Design review of the part built by this model. Coordinates are the model's own, in mm. A direction names the side the tool comes from. Round coordinates to 2 decimals unless told otherwise and drop trailing zeros. Write each loop counter-clockwise with the first axis right and the second up, starting at its lowest first coordinate (ties: lowest second). Pieces come first, ordered by that corner, then holes.
from build123d import *

# Parameters (mm, degrees)
CROQUIS1_W              = 67
CROQUIS1_H              = 51.82
SALIENTE_EXTRUIR1_DEPTH = 70
CORTAR_EXTRUIR1_REACH   = 69
CROQUIS4_W              = 60
CROQUIS4_H              = 30
CORTAR_EXTRUIR2_DEPTH   = 35
CORTAR_EXTRUIR3_REACH   = 69
CROQUIS5_W              = 45
CROQUIS5_H              = 5
CORTAR_EXTRUIR4_REACH   = 53.82
CORTAR_EXTRUIR5_REACH   = 53.82
CROQUIS11_R             = 1.589119195
CROQUIS11_R_2           = 1.628109744
CORTAR_EXTRUIR6_DEPTH   = 6
CROQUIS12_R             = 1.75
CORTAR_EXTRUIR7_DEPTH   = 7
CORTAR_EXTRUIR8_REACH   = 34.863


with BuildPart() as part:
    # Croquis1 → Saliente-Extruir1 (new body)
    with BuildSketch(Plane(origin=(0, 0, 0), x_dir=(0, 0, -1), z_dir=(1, 0, 0))):
        with Locations((33.5, 25.91)):
            Rectangle(CROQUIS1_W, CROQUIS1_H)
    extrude(amount=SALIENTE_EXTRUIR1_DEPTH)

    # Croquis3 → Cortar-Extruir1 (cut, up to next)
    with BuildSketch(Plane.XY, mode=Mode.PRIVATE) as cortar_extruir1_sk1:
        Polygon((70, 0), (20.404370982, 26.370463718), (6.872612509, 51.82), (70, 51.82), align=None)
    cortar_extruir1_tool1 = extrude(cortar_extruir1_sk1.sketch, amount=-CORTAR_EXTRUIR1_REACH, mode=Mode.PRIVATE) & part.part
    add(cortar_extruir1_tool1.solids().sort_by_distance((45.373987, 32.707801, 0))[0], mode=Mode.SUBTRACT)

    # Croquis4 → Cortar-Extruir2 (cut)
    with BuildSketch(Plane(origin=(0, 51.82, 0), x_dir=(1, 0, 0), z_dir=(0, 1, 0))):
        with Locations((30, 33.5)):
            Rectangle(CROQUIS4_W, CROQUIS4_H)
    extrude(amount=-CORTAR_EXTRUIR2_DEPTH, mode=Mode.SUBTRACT)

    # Croquis5 → Cortar-Extruir3 (cut, up to next)
    with BuildSketch(Plane.XY, mode=Mode.PRIVATE) as cortar_extruir3_sk1:
        with Locations((22.5, 2.5)):
            Rectangle(CROQUIS5_W, CROQUIS5_H)
    cortar_extruir3_tool1 = extrude(cortar_extruir3_sk1.sketch, amount=-CORTAR_EXTRUIR3_REACH, mode=Mode.PRIVATE) & part.part
    add(cortar_extruir3_tool1.solids().sort_by_distance((22.5, 2.5, 0))[0], mode=Mode.SUBTRACT)

    # Croquis6 → Cortar-Extruir4 (cut, up to next)
    with BuildSketch(Plane(origin=(0, 51.82, 0), x_dir=(1, 0, 0), z_dir=(0, 1, 0)), mode=Mode.PRIVATE) as cortar_extruir4_sk1:
        Polygon((4.922856145, 67), (0, 64.334655313), (0, 67), align=None)
    cortar_extruir4_tool1 = extrude(cortar_extruir4_sk1.sketch, amount=-CORTAR_EXTRUIR4_REACH, mode=Mode.PRIVATE) & part.part
    add(cortar_extruir4_tool1.solids().sort_by_distance((1.640952, 51.82, -66.111552))[0], mode=Mode.SUBTRACT)

    # Croquis9 → Cortar-Extruir5 (cut, up to next)
    with BuildSketch(Plane(origin=(0, 51.82, 0), x_dir=(1, 0, 0), z_dir=(0, 1, 0)), mode=Mode.PRIVATE) as cortar_extruir5_sk1:
        Polygon((45, 67), (13.626202653, 52.370158031), (1.954435626, 52.832439456), (-4.658833913, 67.014641749), align=None)
    cortar_extruir5_tool1 = extrude(cortar_extruir5_sk1.sketch, amount=-CORTAR_EXTRUIR5_REACH, mode=Mode.PRIVATE) & part.part
    add(cortar_extruir5_tool1.solids().sort_by_distance((15.368059, 51.82, -61.265598))[0], mode=Mode.SUBTRACT)

    # Croquis11 → Cortar-Extruir6 (cut)
    with BuildSketch(Plane.ZY):
        with Locations((-14.75, 23.32)):
            Circle(CROQUIS11_R)
        with Locations((-51.75, 23.32)):
            Circle(CROQUIS11_R_2)
    extrude(amount=-CORTAR_EXTRUIR6_DEPTH, mode=Mode.SUBTRACT)

    # Croquis12 → Cortar-Extruir7 (cut)
    with BuildSketch(Plane.XZ.offset(-5)):
        with Locations((10, -9)):
            Circle(CROQUIS12_R)
        with Locations((35, -9)):
            Circle(CROQUIS12_R)
        with Locations((10, -47.51378034)):
            Circle(CROQUIS12_R)
        with Locations((35, -29)):
            Circle(CROQUIS12_R)
        with Locations((10, -29)):
            Circle(CROQUIS12_R)
        with Locations((35, -54)):
            Circle(CROQUIS12_R)
    extrude(amount=-CORTAR_EXTRUIR7_DEPTH, mode=Mode.SUBTRACT)

    # Croquis14 → Cortar-Extruir8 (cut, up to next)
    with BuildSketch(Plane(origin=(15.428248379, 29.016315039, 0), x_dir=(0.882947593, -0.469471563, 0), z_dir=(0.469471563, 0.882947593, 0)), mode=Mode.PRIVATE) as cortar_extruir8_sk1:
        Polygon((25.978815345, -1.66), (66.698815345, -1.66), (66.698815345, 15.62), align=None)
    cortar_extruir8_tool1 = extrude(cortar_extruir8_sk1.sketch, amount=-CORTAR_EXTRUIR8_REACH, mode=Mode.PRIVATE) & part.part
    add(cortar_extruir8_tool1.solids().sort_by_distance((62.335265, 4.075412, -4.1))[0], mode=Mode.SUBTRACT)


solid = part.part
1) The part is to be moulded in two halves that separate along X. For faces 5 (the face through (0.99, 28.74, -54.9)), 6 (the face through (45, 2, -35)), 7 (the face through (22, 5, -26)), say which applies: pulls with the +X half, pulls with the -X half, needs draft (parallel to the pull), parting line crosses it, or undercut.
2) Add section A-A on z = -14.75. State the section outline as (x, y) points, and give its area (3 significant figures).
3) For line 1 along Z through (x, y) = (35, 7.25); line 2 along Y through (x, z) = (7.5, -19); line 3 along Z through (x, y) = (10, 8.5), list the stretches that pass through material, from the lowest coordinate up.
4) For P1, Ø2.5, axis at y = 23.5, z = -15, coming from the -X side; P2, Ø2, axis at y = 23.32, z = -51.75, coming from the +X side; P3, Ø4, axis at x = 10.5, z = -9.5, coming from the -Y side, all flat-tipped, find the tip position at first contact; note any pin that passes through.
5) Add section C-C on y = 48.5. State the section outline as (x, z) points.
6) Add section D-D on x = 35. State the section outline as (y, z) points.
7) For faces 1 (the face through (10, 31, -18.5)), 2 (the face through (2.958, 23.809, -50.197)), 3 (the face through (26.047, 14.716, -58.162)), 4 (the face through (10, 12, -29)), list the 3-axis set-ups (+Z, -Z, +X, -X, +Y, -Y) from which the entire face can be reached by the end or side of a thin tool; tool diameter is ignored.
8) Add section B-B on y = 23.32. State the section outline as (x, z) points, and give its area (3 significant figures).
Computed:
1. face 5: undercut
1. face 6: pulls with the -X half
1. face 7: needs draft
2. outline: (0, 5) - (45, 5) - (45, 0) - (70, 0) - (20.4, 26.37) - (6.87, 51.82) - (0, 51.82) - (0, 24.91) - (6, 24.91) - (6, 21.73) - (0, 21.73) - close
2. area: 1,300 mm2
3. line 1: z = -62.34 to -55.75, -52.25 to -30.75, -27.25 to -10.75, -7.25 to 0
3. line 2: y = 5 to 16.82
3. line 3: z = -52.51 to -49.26, -45.76 to -30.75, -27.25 to -10.75, -7.25 to 0
4. P1: stops at x = 6
4. P2: stops at x = 28.02
4. P3: stops at y = 5
5. outline: (0, -57.02) - (1.95, -52.83) - (8.64, -52.57) - (8.64, -48.5) - (0, -48.5) - close; (0, -18.5) - (8.64, -18.5) - (8.64, 0) - (0, 0) - close
6. outline: (5, -62.34) - (18.61, -62.34) - (18.61, -48.5) - (16.82, -48.5) - (16.82, -18.5) - (18.61, -18.5) - (18.61, 0) - (5, 0) - (5, -7.25) - (12, -7.25) - (12, -10.75) - (5, -10.75) - (5, -27.25) - (12, -27.25) - (12, -30.75) - (5, -30.75) - (5, -52.25) - (12, -52.25) - (12, -55.75) - (5, -55.75) - close
7. face 1: +X, -X, +Y
7. face 2: -X
7. face 3: -Z, +Y, -Y
7. face 4: -Y
8. outline: (0, -57.02) - (1.7, -53.38) - (0, -53.38) - close; (0, -50.12) - (6, -50.12) - (6, -52.67) - (13.63, -52.37) - (26.14, -58.21) - (26.14, -48.5) - (0, -48.5) - close; (0, -18.5) - (26.14, -18.5) - (26.14, 0) - (0, 0) - (0, -13.16) - (6, -13.16) - (6, -16.34) - (0, -16.34) - close
8. area: 593 mm2
